from build123d import *

# Parameters (mm, degrees)
BOSS_EXTRUDE1_DEPTH = 36
CUT_EXTRUDE1_REACH  = 47.782
SKETCH3_R           = 3.6
CUT_EXTRUDE3_REACH  = 50.982
CUT_EXTRUDE3_START  = -3.2
SKETCH3_4_R         = 5.5
SKETCH3_4_R_2       = 3.6
CUT_EXTRUDE2_REACH  = 47.782
SKETCH4_R           = 3.6
CUT_EXTRUDE4_REACH  = 50.982
CUT_EXTRUDE4_START  = -3.2
SKETCH4_3_R         = 5.5
SKETCH4_3_R_2       = 3.6


with BuildPart() as part:
    # Sketch2 → Boss-Extrude1 (new, symmetric)
    with BuildSketch(Plane(origin=(0, 0, 0), x_dir=(1, 0, 0), z_dir=(0, 1, 0))):
        Polygon((0, 0), (0, 20), (1, 20), (20, 1), (20, 0), align=None)
    extrude(amount=BOSS_EXTRUDE1_DEPTH, both=True)

    # Cut-Extrude1: up to this plane
    cut_extrude1_end = Plane(origin=(1, 36, -20), z_dir=(-0.7071067811865476, 0, 0.7071067811865476))
    # Sketch3 → Cut-Extrude1 (cut, up to the surface)
    with BuildSketch(Plane.XY, mode=Mode.PRIVATE) as cut_extrude1_sk1:
        with Locations((10, 26)):
            Circle(SKETCH3_R)
    cut_extrude1_tool1 = split(extrude(cut_extrude1_sk1.sketch, amount=-CUT_EXTRUDE1_REACH, mode=Mode.PRIVATE), bisect_by=cut_extrude1_end, keep=Keep.BOTH, mode=Mode.PRIVATE)
    add(cut_extrude1_tool1.solids().sort_by_distance((10, 26, 0))[0], mode=Mode.SUBTRACT)
    # Sketch3 → Cut-Extrude1 (cut, up to the surface)
    with BuildSketch(Plane.XY, mode=Mode.PRIVATE) as cut_extrude1_sk2:
        with Locations((10, -26)):
            Circle(SKETCH3_R)
    cut_extrude1_tool2 = split(extrude(cut_extrude1_sk2.sketch, amount=-CUT_EXTRUDE1_REACH, mode=Mode.PRIVATE), bisect_by=cut_extrude1_end, keep=Keep.BOTH, mode=Mode.PRIVATE)
    add(cut_extrude1_tool2.solids().sort_by_distance((10, -26, 0))[0], mode=Mode.SUBTRACT)

    # Cut-Extrude3: up to this plane
    cut_extrude3_end = Plane(origin=(1, 36, -20), z_dir=(-0.7071067811865476, 0, 0.7071067811865476))
    # Sketch3<4> → Cut-Extrude3 (cut, up to the surface)
    with BuildSketch(Plane.XY.offset(CUT_EXTRUDE3_START), mode=Mode.PRIVATE) as cut_extrude3_sk1:
        with Locations((10, 26)):
            Circle(SKETCH3_4_R)
        with Locations((10, 26)):
            Circle(SKETCH3_4_R_2, mode=Mode.SUBTRACT)
    cut_extrude3_tool1 = split(extrude(cut_extrude3_sk1.sketch, amount=-CUT_EXTRUDE3_REACH, mode=Mode.PRIVATE), bisect_by=cut_extrude3_end, keep=Keep.BOTH, mode=Mode.PRIVATE)
    add(cut_extrude3_tool1.solids().sort_by_distance((4.655563, 26, -3.2))[0], mode=Mode.SUBTRACT)
    # Sketch3<4> → Cut-Extrude3 (cut, up to the surface)
    with BuildSketch(Plane.XY.offset(CUT_EXTRUDE3_START), mode=Mode.PRIVATE) as cut_extrude3_sk2:
        with Locations((10, -26)):
            Circle(SKETCH3_4_R)
        with Locations(Location((10, -26, 0), (0, 0, 180))):
            Circle(SKETCH3_4_R_2, mode=Mode.SUBTRACT)
    cut_extrude3_tool2 = split(extrude(cut_extrude3_sk2.sketch, amount=-CUT_EXTRUDE3_REACH, mode=Mode.PRIVATE), bisect_by=cut_extrude3_end, keep=Keep.BOTH, mode=Mode.PRIVATE)
    add(cut_extrude3_tool2.solids().sort_by_distance((4.655563, -26, -3.2))[0], mode=Mode.SUBTRACT)

    # Cut-Extrude2: up to this face of the body (flat: up to its plane)
    cut_extrude2_end = Plane(part.part.faces().sort_by_distance((10.58067787, 0, -10.41932213))[0])
    # Sketch4 → Cut-Extrude2 (cut, up to the picked face)
    with BuildSketch(Plane.ZY, mode=Mode.PRIVATE) as cut_extrude2_sk1:
        with Locations((-10, 26)):
            Circle(SKETCH4_R)
    cut_extrude2_tool1 = split(extrude(cut_extrude2_sk1.sketch, amount=-CUT_EXTRUDE2_REACH, mode=Mode.PRIVATE), bisect_by=cut_extrude2_end, keep=Keep.BOTH, mode=Mode.PRIVATE)
    # Sketch4 → Cut-Extrude2 (cut, up to the picked face)
    with BuildSketch(Plane.ZY, mode=Mode.PRIVATE) as cut_extrude2_sk2:
        with Locations((-10, -26)):
            Circle(SKETCH4_R)
    cut_extrude2_tool2 = split(extrude(cut_extrude2_sk2.sketch, amount=-CUT_EXTRUDE2_REACH, mode=Mode.PRIVATE), bisect_by=cut_extrude2_end, keep=Keep.BOTH, mode=Mode.PRIVATE)
    add(cut_extrude2_tool1.solids().sort_by(Axis((0, 26, -10), (1, 0, 0)))[0], mode=Mode.SUBTRACT)
    add(cut_extrude2_tool2.solids().sort_by(Axis((0, -26, -10), (1, 0, 0)))[0], mode=Mode.SUBTRACT)

    # Cut-Extrude4: up to this plane
    cut_extrude4_end = Plane(origin=(1, 36, -20), z_dir=(-0.7071067811865476, 0, 0.7071067811865476))
    # Sketch4<3> → Cut-Extrude4 (cut, up to the surface)
    with BuildSketch(Plane.ZY.offset(CUT_EXTRUDE4_START), mode=Mode.PRIVATE) as cut_extrude4_sk1:
        with Locations((-10, 26)):
            Circle(SKETCH4_3_R)
        with Locations((-10, 26)):
            Circle(SKETCH4_3_R_2, mode=Mode.SUBTRACT)
    cut_extrude4_tool1 = split(extrude(cut_extrude4_sk1.sketch, amount=-CUT_EXTRUDE4_REACH, mode=Mode.PRIVATE), bisect_by=cut_extrude4_end, keep=Keep.BOTH, mode=Mode.PRIVATE)
    add(cut_extrude4_tool1.solids().sort_by_distance((3.2, 26, -15.344437))[0], mode=Mode.SUBTRACT)
    # Sketch4<3> → Cut-Extrude4 (cut, up to the surface)
    with BuildSketch(Plane.ZY.offset(CUT_EXTRUDE4_START), mode=Mode.PRIVATE) as cut_extrude4_sk2:
        with Locations(Location((-10, -26, 0), (0, 0, 270))):
            Circle(SKETCH4_3_R)
        with Locations((-10, -26)):
            Circle(SKETCH4_3_R_2, mode=Mode.SUBTRACT)
    cut_extrude4_tool2 = split(extrude(cut_extrude4_sk2.sketch, amount=-CUT_EXTRUDE4_REACH, mode=Mode.PRIVATE), bisect_by=cut_extrude4_end, keep=Keep.BOTH, mode=Mode.PRIVATE)
    add(cut_extrude4_tool2.solids().sort_by_distance((3.2, -20.655563, -10))[0], mode=Mode.SUBTRACT)


solid = part.part
CAD build for the part. Positions are in the model's coordinates, mm. A direction names the side the tool comes from. Round coordinates to 2 decimals unless told otherwise and drop trailing zeros. Order: outer loops, then holes, each group sorted by start corner. A loop starts at its lowest first (then second) coordinate and runs counter-clockwise, first axis right, second up. Notation, with made-up numbers: (-13, -2.75) -> (26, -2.75) arc R33 ccw to (26, 31.25) -> close; hole circle Ø4 at (-2, 27). An arc over 180 degrees is marked (long way). Write item = value, one per line. Start each with the question number.
(1) Cut at C-C, the plane y = 6. List the corners of the cut face in (x, z).
(2) Cut at B-B, the plane x = 7.5. List the corners of the cut face in (y, z).
(3) Cut at D-D, the plane z = -18. List the corners of the cut face in (x, y), then the cut area to 3 significant figures.
(4) Probe line 1 (Y direction, x = 10, z = -2.15); line 2 (Y direction, x = 9, z = -8.75); line 3 (X direction, y = 26, z = -5.75). List the from-to ranges inside material, lowest first. Write a range as [from, to].
(5) Pull direction Y, two halves, no side cores. Call faces 4 (the flat face through (10, 1, -11)), 5 (the flat face through (8, 36, -8)), 6 (the cylindrical face through (5.041, -20.505, -9.758)): released by +Y, released by -Y, zero draft, split by the parting line, or undercut.
(6) Cut at A-A, the plane y = 26. List the corners of the cut face in (x, z).
(7) Pin check, flat tips, straight feed: P1, Ø3.5, axis at x = 7.5, y = 27.5, coming from the -Z side; P2, Ø9, axis at y = 28.5, z = -12, coming from the +X side; P3, Ø6.5, axis at x = 10, y = 26, coming from the +Z side; P4, Ø12, axis at y = -22.5, z = -6.5, coming from the +X side. Stop position of each tip, or through.
(8) Which spindle directions (+Z, -Z, +X, -X, +Y, -Y) get a long thin tool onto all of the face, cutting with end or side? Do faces 1 (the cylindrical face through (1.578, -24.919, -6.566)), 2 (the flat face through (3.2, -27, -14)), 3 (the flat face through (14, -27, -3.2)). Say none if no direction does.
Model answer:
q1.outline = (0, -20) -> (1, -20) -> (20, -1) -> (20, 0) -> (0, 0) -> close
q2.outline = (-36, -13.5) -> (-30.9, -13.5) -> (-30.9, -12.5) arc R5.5 cw to (-30.9, -7.5) -> (-30.9, -3.2) -> (-28.59, -3.2) -> (-28.59, 0) -> (-36, 0) -> close; (-23.41, -3.2) -> (-21.1, -3.2) -> (-21.1, -7.5) arc R5.5 cw to (-21.1, -12.5) -> (-21.1, -13.5) -> (21.1, -13.5) -> (21.1, -12.5) arc R5.5 cw to (21.1, -7.5) -> (21.1, -3.2) -> (23.41, -3.2) -> (23.41, 0) -> (-23.41, 0) -> close; (28.59, -3.2) -> (30.9, -3.2) -> (30.9, -7.5) arc R5.5 cw to (30.9, -12.5) -> (30.9, -13.5) -> (36, -13.5) -> (36, 0) -> (28.59, 0) -> close
q3.outline = (0, -36) -> (3, -36) -> (3, 36) -> (0, 36) -> close
q3.area = 216 mm2
q4.line_1 = [-36, -29.6], [-22.4, 22.4], [29.6, 36]
q4.line_2 = [-36, -31.41], [-20.59, 20.59], [31.41, 36]
q4.line_3 = [0, 3.2]
q5.face_4 = zero draft
q5.face_5 = released by +Y
q5.face_6 = undercut
q6.outline = (0, -20) -> (1, -20) -> (4.5, -16.5) -> (4.5, -15.5) -> (3.2, -15.5) -> (3.2, -13.6) -> (0, -13.6) -> close; (0, -6.4) -> (3.2, -6.4) -> (3.2, -4.5) -> (4.5, -4.5) -> (4.5, -3.2) -> (6.4, -3.2) -> (6.4, 0) -> (0, 0) -> close; (13.6, -3.2) -> (15.5, -3.2) -> (15.5, -4.5) -> (16.5, -4.5) -> (20, -1) -> (20, 0) -> (13.6, 0) -> close
q7.P1 = -3.2
q7.P2 = 12.54
q7.P3 = through
q7.P4 = 20
q8.face_1 = +X, -X
q8.face_2 = +X
q8.face_3 = -Z
